Could you check a few things on this model? Use its own coordinates, in mm. A direction names the side the tool comes from. Give positions to 0.01 mm unless a question says otherwise; leave off trailing zeros. Order: outer loops, then holes, each group sorted by start corner. A loop starts at its lowest first (then second) coordinate and runs counter-clockwise, first axis right, second up. Notation, with made-up numbers: (24, 51) -> (83, 51) arc R19 ccw to (83, 87) -> close; hole circle Ø1 at (-24, 8). An arc over 180 degrees is marked (long way). Use one line per item in the form item = value. Start each with the question number.
from build123d import *

# Parameters (mm, degrees)
F0_R      = 17.145
F0_R_2    = 13.97
F1_DEPTH  = 0.762
F0_R_3    = 12.065
F2_DEPTH  = 0.508
F3_DEPTH  = 0.254
F0_R_4    = 0.381
F5_DEPTH  = 0.381
F6_DEPTH  = 0.508
F7_DEPTH  = 1.016
F8_R      = 1.905
F9_DEPTH  = 25.4
F10_DEPTH = 3.048
F11_R     = 3.048
F11_R_2   = 1.905
F12_DEPTH = 8.128
F13_R     = 13.97
F13_R_2   = 12.065
F14_DEPTH = 0.762
F15_DEPTH = 1.27


# Not quite as in the source:
# - the program builds the solid bodies; features that only make, move or delete a surface that nothing else refers to are left out


with BuildPart() as f1:
    # F0 (on Front) → F1 (new body)
    with BuildSketch(Plane.XZ):
        Circle(F0_R)
        Circle(F0_R_2, mode=Mode.SUBTRACT)
    extrude(amount=F1_DEPTH)

    # F0 (on Front) → F2 (join)
    with BuildSketch(Plane.XZ):
        Circle(F0_R_2)
        Circle(F0_R_3, mode=Mode.SUBTRACT)
    extrude(amount=F2_DEPTH)

    # F0 (on Front) → F3 (join)
    with BuildSketch(Plane.XZ):
        Circle(F0_R_3)
        with BuildLine():
            ThreePointArc((0, 5.715), (4.0411152545, 4.0411152545), (5.715, 0))
            ThreePointArc((5.715, 0), (-4.0411152545, -4.0411152545), (0, 5.715))
        make_face(mode=Mode.SUBTRACT)
    extrude(amount=F3_DEPTH)

    # F0 (on Front) → F5 (join)
    with BuildSketch(Plane.XZ):
        with BuildLine():
            ThreePointArc((0, 5.715), (-4.0411152545, -4.0411152545), (5.715, 0))
            ThreePointArc((5.715, 0), (4.0411152545, 4.0411152545), (0, 5.715))
        make_face()
        with Locations((-1.2134722805, -3.1998572434)):
            Circle(F0_R_4, mode=Mode.SUBTRACT)
        with Locations((-2.8625485942, -1.8754777789)):
            Circle(F0_R_4, mode=Mode.SUBTRACT)
        with Locations((0.8991092, -3.302)):
            Circle(F0_R_4, mode=Mode.SUBTRACT)
        with Locations((2.6682615257, -2.1428909875)):
            Circle(F0_R_4, mode=Mode.SUBTRACT)
        with Locations((3.4182286394, -0.1652704519)):
            Circle(F0_R_4, mode=Mode.SUBTRACT)
        with Locations((-3.4182286394, 0.1652704519)):
            Circle(F0_R_4, mode=Mode.SUBTRACT)
        with Locations((-2.6682615257, 2.1428909875)):
            Circle(F0_R_4, mode=Mode.SUBTRACT)
        with Locations((-0.8991092, 3.302)):
            Circle(F0_R_4, mode=Mode.SUBTRACT)
        with BuildLine():
            ThreePointArc((0.889, 0), (-0.6286179285, -0.6286179285), (0, 0.889))
            ThreePointArc((0, 0.889), (0.6286179285, 0.6286179285), (0.889, 0))
        make_face(mode=Mode.SUBTRACT)
        with Locations((2.8625485942, 1.8754777789)):
            Circle(F0_R_4, mode=Mode.SUBTRACT)
        with BuildLine():
            ThreePointArc((1.5944722805, 3.1998572434), (1.161927001, 2.8223601121), (0.8464193452, 3.302))
            ThreePointArc((0.8464193452, 3.302), (1.2650175599, 3.5773543747), (1.5944722805, 3.1998572434))
        make_face(mode=Mode.SUBTRACT)
    extrude(amount=F5_DEPTH)

    # F0 (on Front) → F6 (join)
    with BuildSketch(Plane.XZ):
        with Locations((-0.8991092, 3.302)):
            Circle(F0_R_4)
        with BuildLine():
            ThreePointArc((1.5944722805, 3.1998572434), (1.2650175599, 3.5773543747), (0.8464193452, 3.302))
            ThreePointArc((0.8464193452, 3.302), (1.161927001, 2.8223601121), (1.5944722805, 3.1998572434))
        make_face()
        with Locations((-2.6682615257, 2.1428909875)):
            Circle(F0_R_4)
        with Locations((2.8625485942, 1.8754777789)):
            Circle(F0_R_4)
        with Locations((3.4182286394, -0.1652704519)):
            Circle(F0_R_4)
        with Locations((-1.2134722805, -3.1998572434)):
            Circle(F0_R_4)
        with Locations((-2.8625485942, -1.8754777789)):
            Circle(F0_R_4)
        with Locations((-3.4182286394, 0.1652704519)):
            Circle(F0_R_4)
        with Locations((2.6682615257, -2.1428909875)):
            Circle(F0_R_4)
        with Locations((0.8991092, -3.302)):
            Circle(F0_R_4)
    extrude(amount=F6_DEPTH)

    # F0 (on Front) → F7 (join)
    with BuildSketch(Plane.XZ):
        with BuildLine():
            ThreePointArc((0.889, 0), (0.6286179285, 0.6286179285), (0, 0.889))
            ThreePointArc((0, 0.889), (-0.6286179285, -0.6286179285), (0.889, 0))
        make_face()
    extrude(amount=F7_DEPTH)

    # F8 (on face) → F9 (cut)
    with BuildSketch(Plane.XZ.offset(0.254)):
        with Locations((-2.1587662638, 8.89)):
            Circle(F8_R)
        with Locations((-6.9718894872, 5.923270107)):
            Circle(F8_R)
        with Locations((-9.1219878923, 0.6940523577)):
            Circle(F8_R)
        with Locations((-7.7877969675, -4.8002698023)):
            Circle(F8_R)
        with Locations((-3.4789322986, -8.461052053)):
            Circle(F8_R)
        with Locations((2.1587662638, -8.89)):
            Circle(F8_R)
        with Locations((6.9718894872, -5.923270107)):
            Circle(F8_R)
        with Locations((9.1219878923, -0.6940523577)):
            Circle(F8_R)
        with Locations((7.7877969675, 4.8002698023)):
            Circle(F8_R)
        with Locations((3.4789322986, 8.461052053)):
            Circle(F8_R)
    extrude(amount=-F9_DEPTH, mode=Mode.SUBTRACT)

    # F10 (add): a face of the model
    f10_faces = [f1.faces().sort_by_distance(p)[0] for p in [
        (0, 0, 0),
    ]]
    extrude(f10_faces, amount=F10_DEPTH)

    # F11 (on face) → F12 (join)
    with BuildSketch(Plane(origin=(0, 3.048, 0), x_dir=(-1, 0, 0), z_dir=(0, 1, 0))):
        Circle(F11_R)
        Circle(F11_R_2, mode=Mode.SUBTRACT)
    extrude(amount=F12_DEPTH)

    # F13 (on face) → F14 (cut)
    with BuildSketch(Plane(origin=(0, 3.048, 0), x_dir=(-1, 0, 0), z_dir=(0, 1, 0))):
        Circle(F13_R)
        Circle(F13_R_2, mode=Mode.SUBTRACT)
    extrude(amount=-F14_DEPTH, mode=Mode.SUBTRACT)

    # F15 (cut): a face of the model
    f15_faces = [f1.faces().sort_by_distance(p)[0] for p in [
        (11.7237502674, 3.048, 0),
    ]]
    extrude(f15_faces, amount=-F15_DEPTH, mode=Mode.SUBTRACT)


solid = f1.part
(1) We'd pull the mould along Z, two halves only. Please class faces 4 (the flat face through (-6, 3.048, -13)), 5 (the cylindrical face through (7.54, 0.75, 6.69)): pulls with the +Z half, pulls with the -Z half, needs draft (parallel to the pull), parting line crosses it, or undercut.
(2) Imagine slicing it at A-A (z = -8.89). Write out the boundary of the cut face in (x, y), plus the area to 3 significant figures.
(3) Imagine slicing it at B-B (x = 8). Give the number of separate pieces and of enclosed holes in the cut face, plus the area to 3 significant figures.
(4) Please list where these lines run through material, in increasing order: probe 1 along Z at (x, y) = (0, -0.35) (3 decimals); probe 2 along Y at (x, z) = (-6.5, 8.5); probe 3 along X at (y, z) = (2.75, 12.5).
(5) Imagine slicing it at C-C (y = 8.75). Write out the boundary of the cut face in (x, z) (3 decimals), plus the area to 3 significant figures.
(6) Which directions (+Z, -Z, +X, -X, +Y, -Y) give clear straight access to the entire face, cutting with the end or side of a thin tool? Please do faces 1 (the cylindrical face through (0.4, 6.54, 3.02)), 2 (the flat face through (1.2, -0.381, 0.1)), 3 (the cylindrical face through (1.91, 0.75, -7)).
(7) Imagine slicing it at D-D (z = 13). Write out the boundary of the cut face in (x, y), plus the area to 3 significant figures.
(8) I'm going to push flat-ended pins straight in: pin 1 Ø2 at (y, z) = (0.5, 11) entering from +X; pin 2 Ø0.8 at (x, z) = (2.5, 1.5) entering from -Y; pin 3 Ø5 at (x, y) = (-3, 1.5) entering from -Z. Where does each tip first touch, or does it pass through?
Calculated:
q1.face_4 = needs draft
q1.face_5 = undercut
q2.outline = (-14.66, -0.76) -> (-10.78, -0.76) -> (-10.78, -0.51) -> (-8.16, -0.51) -> (-8.16, -0.25) -> (-5.34, -0.25) -> (-5.34, 1.78) -> (-8.16, 1.78) -> (-8.16, 2.29) -> (-10.78, 2.29) -> (-10.78, 3.05) -> (-14.66, 3.05) -> close; (-1.62, -0.25) -> (0.25, -0.25) -> (0.25, 1.78) -> (-1.62, 1.78) -> close; (4.06, -0.25) -> (8.16, -0.25) -> (8.16, -0.51) -> (10.78, -0.51) -> (10.78, -0.76) -> (14.66, -0.76) -> (14.66, 3.05) -> (10.78, 3.05) -> (10.78, 2.29) -> (8.16, 2.29) -> (8.16, 1.78) -> (4.06, 1.78) -> close
q2.area = 62.1 mm2
q3.separate_pieces = 4
q3.enclosed_holes = 0
q3.area = 58.0 mm2
q4.probe_1 = -17.145 to -12.065, -5.715 to 5.715, 12.065 to 17.145
q4.probe_2 = -0.25 to 1.78
q4.probe_3 = -11.73 to -6.24, 6.24 to 11.73
q5.outline = circle Ø6.096 at (0, 0); hole circle Ø3.81 at (0, 0)
q5.area = 17.8 mm2
q6.face_1 = +Y
q6.face_2 = -Y
q6.face_3 = +Y, -Y
q7.outline = (-11.18, -0.76) -> (-5.11, -0.76) -> (-5.11, -0.51) -> (5.11, -0.51) -> (5.11, -0.76) -> (11.18, -0.76) -> (11.18, 3.05) -> (5.11, 3.05) -> (5.11, 2.29) -> (-5.11, 2.29) -> (-5.11, 3.05) -> (-11.18, 3.05) -> close
q7.area = 74.8 mm2
q8.pin_1 = 13.93
q8.pin_2 = -0.51
q8.pin_3 = -17.14
